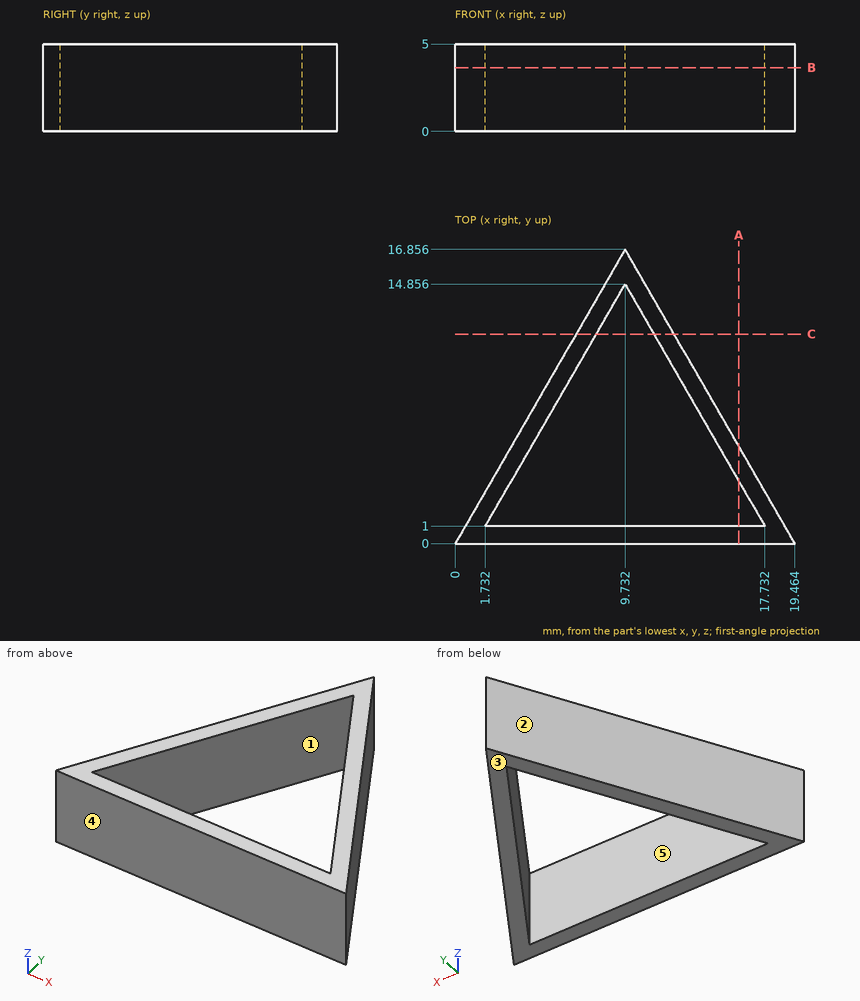
The figure shows three views and two pictorial views of one solid part (mm, origin at its lowest corner). Answer the questions. A direction names the side the tool comes from. Coordinates: 2 decimals unless noted, no trailing zeros. Write each loop counter-clockwise with the first axis right and the second up, starting at its lowest first coordinate (ties: lowest second). Pieces come first, ordered by that corner, then holes.
1. For the marked faces 4 and 5, determine the directions among +Z, -Z, +X, -X, +Y, -Y from which every point of the face is accessible in a straight line to the end or side of a thin tool.
Results list:
face 4: +Z, -Z, +X, -X, -Y
face 5: +Z, -Z
2. The part is cut by section C-C, the plane y = 12. Write down the section's boundary in (x, z).
Results list:
outline: (6.93, 0) - (8.08, 0) - (8.08, 5) - (6.93, 5) - close; (11.38, 0) - (12.54, 0) - (12.54, 5) - (11.38, 5) - close
3. The part is cut by section B-B, the plane z = 3.65. Write down the section's boundary in (x, y) (1 decimal).
Results list:
outline: (0, 0) - (19.5, 0) - (9.7, 16.9) - close; hole (1.7, 1) - (17.7, 1) - (9.7, 14.9) - close
4. For a pull along X with two mould halves and no side action, classify the marked faces 1, 2 and 3 as +X half, -X half, draft (parallel to the pull), parting line (faces both ways), or undercut.
Results list:
face 1: undercut
face 2: -X half
face 3: draft
5. The part is cut by section A-A, the plane x = 16.25. Write down the section's boundary in (y, z).
Results list:
outline: (0, 0) - (1, 0) - (1, 5) - (0, 5) - close; (3.57, 0) - (5.57, 0) - (5.57, 5) - (3.57, 5) - close
6. Consider line 1 along X through (y, z) = (13, 4.55) (1 decimal); line 2 along Y through (x, z) = (13.75, 0.8) (1 decimal); line 3 along X through (y, z) = (9.5, 4.5) (1 decimal). Determine where each line is inside the solid, lowest interval first.
Results list:
line 1: x = 7.5 to 8.7, 10.8 to 12
line 2: y = 0 to 1, 7.9 to 9.9
line 3: x = 5.5 to 6.6, 12.8 to 14
7. Flat-ended cylindrical pins translate along their axes: pin 1 (1 mm diameter, centred on x = 5, y = 2, fed in from -Z); pin 2 (1 mm diameter, centred on y = 13.5, z = 3, fed in from +X); pin 3 (3 mm diameter, centred on y = 10.5, z = 0.5, fed in from +X); pin 4 (1.5 mm diameter, centred on x = 11, z = 3, fed in from +Y). Find the tip coordinate at first contact, or state that the pin passes through.
Results list:
pin 1: passes through
pin 2: stops at x = 11.96
pin 3: stops at x = 14.27
pin 4: stops at y = 15.96
